Source: CAD feature listing. Evaluate the final solid. Frame: model axes, mm. Coordinates: 2 decimals unless noted, no trailing zeros. Order: outer loops, then holes, each group sorted by start corner. A loop starts at its lowest first (then second) coordinate and runs counter-clockwise, first axis right, second up. Notation, with made-up numbers: (31, -2) - (76, -2) arc R23 ccw to (76, 18) - close; hole circle Ø2 at (-3, 0.5). An arc over 180 degrees is marked (long way). One line per question, with ' | ' between items.
from build123d import *

# Parameters (mm, degrees)
SKETCH1_R      = 1.25
EXTRUDE1_DEPTH = 16.5
CHAMFER1_SIZE  = 0.2
SKETCH2_R      = 1.25
SKETCH2_R_2    = 0.75
EXTRUDE2_DEPTH = 1.5
FILLET1_R      = 0.25


with BuildPart() as part:
    # Sketch1 → Extrude1 (new body)
    with BuildSketch(Plane(origin=(0, 0, 0), x_dir=(1, 0, 0), z_dir=(0, 1, 0))):
        with Locations(Location((0, 0, 0), (0, 0, 270))):  # turned: the seam where the file's is
            Circle(SKETCH1_R)
    extrude(amount=-EXTRUDE1_DEPTH)

    # Chamfer1
    chamfer1_edges = [part.edges().sort_by_distance(p)[0] for p in [
        (0, 0, -1.25),
        (0, -16.5, -1.25),
    ]]
    chamfer(chamfer1_edges, length=CHAMFER1_SIZE)

    # Sketch2 → Extrude2 (cut)
    with BuildSketch(Plane.XZ.offset(2.5)):
        with Locations(Location((0, 0, 0), (0, 0, 90))):  # turned: the seam where the file's is
            Circle(SKETCH2_R)
        with Locations(Location((0, 0, 0), (0, 0, 270))):  # turned: the seam where the file's is
            Circle(SKETCH2_R_2, mode=Mode.SUBTRACT)
    extrude(amount=-EXTRUDE2_DEPTH, mode=Mode.SUBTRACT)

    # Fillet1
    fillet1_edges = [part.edges().sort_by_distance(p)[0] for p in [
        (0, -1, 0.75),
        (0, -2.5, 0.75),
    ]]
    fillet(fillet1_edges, radius=FILLET1_R)


solid = part.part
(1) Material intervals for L1, parallel to Z at x = -1, y = -13; L2, parallel to X at y = -3, z = 0.75, sorted ascending. Write a range as from..to.
Taken from the geometry:
L1: z = -0.75..0.75 | L2: x = -1..1
(2) Cut plane A-A (z = 0). Return the cut outline in (x, y), and give its area (3 significant figures).
Taken from the geometry:
outline: (-1.25, -16.3) - (-1.05, -16.5) - (1.05, -16.5) - (1.25, -16.3) - (1.25, -2.5) - (1, -2.5) arc R0.25 cw to (0.75, -2.25) - (0.75, -1.25) arc R0.25 cw to (1, -1) - (1.25, -1) - (1.25, -0.2) - (1.05, 0) - (-1.05, 0) - (-1.25, -0.2) - (-1.25, -1) - (-1, -1) arc R0.25 cw to (-0.75, -1.25) - (-0.75, -2.25) arc R0.25 cw to (-1, -2.5) - (-1.25, -2.5) - close | area: 39.7 mm²
(3) Cut plane C-C (y = -13.75). Return the cut outline in (x, z).
Taken from the geometry:
outline: circle Ø2.5 at (0, 0)
(4) Pull-direction query (Y, two-part tool) for faces 1 (the cylindrical face through (0.225, -1.757, -0.715)), 2 (the cylindrical face through (-1.22, -0.59, -0.27)), 3 (the flat face through (0, 0, 0)); classes: pulls with the +Y half, pulls with the -Y half, needs draft (parallel to the pull), parting line crosses it, or undercut.
Taken from the geometry:
face 1: undercut | face 2: needs draft | face 3: pulls with the +Y half
(5) Cut plane B-B (x = 0). Return the cut outline in (y, z).
Taken from the geometry:
outline: (-16.5, -1.05) - (-16.3, -1.25) - (-2.5, -1.25) - (-2.5, -1) arc R0.25 cw to (-2.25, -0.75) - (-1.25, -0.75) arc R0.25 cw to (-1, -1) - (-1, -1.25) - (-0.2, -1.25) - (0, -1.05) - (0, 1.05) - (-0.2, 1.25) - (-1, 1.25) - (-1, 1) arc R0.25 cw to (-1.25, 0.75) - (-2.25, 0.75) arc R0.25 cw to (-2.5, 1) - (-2.5, 1.25) - (-16.3, 1.25) - (-16.5, 1.05) - close
(6) Cut plane D-D (y = -2). Return the cut outline in (x, z), and give its area (3 significant figures).
Taken from the geometry:
outline: circle Ø1.5 at (0, 0) | area: 1.77 mm²
